```python
from build123d import *

# Parameters (mm, degrees)
BOSS_EXTRUDE1_DEPTH = 20
SKETCH2_R           = 1.5
CUT_EXTRUDE1_DEPTH  = 6.5
SKETCH4_W           = 3.5
SKETCH4_H           = 10
BOSS_EXTRUDE2_DEPTH = 20
BOSS_EXTRUDE3_DEPTH = 3.5
SKETCH6_R           = 1.5
CUT_EXTRUDE2_DEPTH  = 20


with BuildPart() as part:
    # Sketch1 → Boss-Extrude1 (new body)
    with BuildSketch(Plane.XY):
        with BuildLine():
            Line((-10, 0), (10, 0))
            Line((10, 0), (10, -14.5))
            Line((10, -14.5), (2.672015421, -14.5))
            Line((2.672015421, -14.5), (2.672015421, -12.5))
            Line((2.672015421, -12.5), (5.422015421, -12.5))
            Line((5.422015421, -12.5), (5.422015421, -10.5))
            Line((5.422015421, -10.5), (2.672015421, -10.5))
            Line((2.672015421, -10.5), (2.672015421, -6.5))
            Line((2.672015421, -6.5), (-5.327984579, -6.5))
            Line((-5.327984579, -6.5), (-5.327984579, -10.5))
            Line((-5.327984579, -10.5), (-8.077984579, -10.5))
            Line((-8.077984579, -10.5), (-8.077984579, -12.5))
            Line((-8.077984579, -12.5), (-5.327984579, -12.5))
            Line((-5.327984579, -12.5), (-5.327984579, -14.5))
            Line((-5.327984579, -14.5), (-8.5, -14.5))
            Line((-8.5, -14.5), (-8.5, -16))
            Line((-8.5, -16), (-12, -16))
            add(Edge.make_bspline(
                [(-10, 0), (-12.576646285, -7.740566288), (-12.284280687, -10.492382976), (-12, -16)],
                knots=[0, 0, 0, 0, 1, 1, 1, 1], degree=3))
        make_face()
    extrude(amount=BOSS_EXTRUDE1_DEPTH)

    # Sketch2 → Cut-Extrude1 (cut)
    with BuildSketch(Plane.XZ.offset(6.5)):
        with Locations((-1.327984579, 15)):
            Circle(SKETCH2_R)
        with Locations((-1.327984579, 5)):
            Circle(SKETCH2_R)
    extrude(amount=-CUT_EXTRUDE1_DEPTH, mode=Mode.SUBTRACT)

    # Sketch4 → Boss-Extrude2 (add)
    with BuildSketch(Plane.XZ.offset(16)):
        with Locations((-10.25, 10)):
            Rectangle(SKETCH4_W, SKETCH4_H)
    extrude(amount=BOSS_EXTRUDE2_DEPTH)

    # Sketch5 → Boss-Extrude3 (add)
    with BuildSketch(Plane.ZY.offset(12)):
        with BuildLine():
            Line((5, -36), (15, -36))
            ThreePointArc((15, -36), (10, -41), (5, -36))
        make_face()
    extrude(amount=-BOSS_EXTRUDE3_DEPTH)

    # Sketch6 → Cut-Extrude2 (cut)
    with BuildSketch(Plane.ZY.offset(12)):
        with Locations((10, -36)):
            Circle(SKETCH6_R)
    extrude(amount=-CUT_EXTRUDE2_DEPTH, mode=Mode.SUBTRACT)


solid = part.part
```
Build history of the part. All positions in model axes, mm. A direction names the side the tool comes from. Give positions to 0.01 mm unless a question says otherwise; leave off trailing zeros. Loops run counter-clockwise (first coordinate to the right, second up) from the corner with the lowest first, then second, coordinate; pieces in that order, holes last. Notation, with made-up numbers: (-20, 52) -> (21, 52) arc R22 cw to (21, 91) -> close; hole circle Ø9 at (8.25, 58). An arc over 180 degrees is marked (long way). One line per question, with ' | ' between items. Start each with the question number.
1) 3-axis set-ups, long thin cutter, end or side, ignore diameter. For faces 1 (the flat face through (6, -14.5, 10)), 2 (the flat face through (2.672, -14, 10)), 3 (the flat face through (-7, -12.5, 10)): which of +Z, -Z, +X, -X, +Y, -Y reach the whole face in a straight line?
2) Cut at C-C (y = -24). Give the cut face in (x, z).
3) Probe L1, parallel to X at y = -12, z = 4.25; L2, parallel to Z at x = -1.5, y = -5; L3, parallel to Y at x = 5.25, z = 1.75. List the from-to ranges inside material, lowest first.
4) Cut at B-B (x = 2). Give the cut face in (y, z).
5) Pin check, flat tips, straight feed: pin 1 (10 mm diameter, centred on x = 0, y = -28.5, fed in from +Z) (3 decimals); pin 2 (3 mm diameter, centred on x = -9.5, z = 18.5, fed in from -Y); pin 3 (2 mm diameter, centred on y = -7, z = 4, fed in from -X); pin 4 (5 mm diameter, centred on x = -6.5, y = -22.5, fed in from +Z). Stop position of each tip, or through.
6) Cut at D-D (y = -5). Count the separate pieces of the cut face and the enclosed holes in it, plus the area to 3 significant figures.
7) Cut at A-A (x = -6.25). Give the cut face in (y, z), plus the area to 3 significant figures.
8) Two-plate mould, pull along Y, no slides. Class faces 4 (the flat face through (5.422, -12, 10)), 5 (the flat face through (0, 0, 10)), 6 (the flat face through (-10, -26, 15)): released by +Y, released by -Y, zero draft, split by the parting line, or undercut.
Return value:
1) face 1: +Z, -Z, +X, -Y | face 2: +Z, -Z, -Y | face 3: +Z, -Z
2) outline: (-12, 5) -> (-8.5, 5) -> (-8.5, 15) -> (-12, 15) -> close
3) L1: -12.18 to -8.08, 5.42 to 10 | L2: 0 to 3.51, 6.49 to 13.51, 16.49 to 20 | L3: -14.5 to -12.5, -10.5 to 0
4) outline: (-6.5, 0) -> (0, 0) -> (0, 20) -> (-6.5, 20) -> close
5) pin 1: through | pin 2: y = -16 | pin 3: x = -11.98 | pin 4: z = 15
6) separate pieces: 1 | enclosed holes: 2 | area: 415 mm^2
7) outline: (-14.5, 0) -> (-12.5, 0) -> (-12.5, 20) -> (-14.5, 20) -> close; (-10.5, 0) -> (0, 0) -> (0, 20) -> (-10.5, 20) -> close | area: 250 mm^2
8) face 4: undercut | face 5: released by +Y | face 6: zero draft
